The listing builds one solid part. Answer for the finished solid, in the listing's coordinates (mm). Face numbers are marked on the shaded views. A direction names the side the tool comes from. Round coordinates to 2 decimals unless told otherwise and drop trailing zeros. Write each loop counter-clockwise with the first axis right and the second up, starting at its lowest first coordinate (ties: lowest second). Pieces come first, ordered by that corner, then holes. Notation, with made-up numbers: M 14,-17.75 L 26,-17.75 A23 cw 26,-5.75 Z; hole C -9,-1 d4. An arc over 180 degrees is marked long. Write each question's results on one line, items separated by ' | '.
from build123d import *

# Parameters (mm, degrees)
F1_DEPTH       = 25
F2_R           = 20
F3_R           = 5
F5_D           = 6.7564
F5_DEPTH       = 15
F5_CSINK_D     = 13.4874
F5_CSINK_ANGLE = 82
F5_TIP         = 2.0298273432
F6_R           = 2


with BuildPart() as f1:
    # F0 (on Front) → F1 (new body)
    with BuildSketch(Plane.XZ):
        Polygon((-70.8, 12.7), (-102.55, 12.7), (-102.55, 0), (102.55, 0), (102.55, 12.7), (70.8, 12.7), (50.8, 12.7), (-50.8, 12.7), align=None)
        with BuildLine():
            ThreePointArc((70.8, 12.7), (0, 83.5), (-70.8, 12.7))
            Line((-70.8, 12.7), (-50.8, 12.7))
            ThreePointArc((-50.8, 12.7), (0, 63.5), (50.8, 12.7))
            Line((50.8, 12.7), (70.8, 12.7))
        make_face()
    extrude(amount=F1_DEPTH)

    # F2
    f2_edges = [f1.edges().sort_by_distance(p)[0] for p in [
        (50.8, -12.5, 12.7),
        (-50.8, -12.5, 12.7),
    ]]
    fillet(f2_edges, radius=F2_R)

    # F3
    f3_edges = [f1.edges().sort_by_distance(p)[0] for p in [
        (70.8, -12.5, 12.7),
        (-70.8, -12.5, 12.7),
    ]]
    fillet(f3_edges, radius=F3_R)

    # F5
    with Locations(Plane.XY.offset(12.7)):
        with Locations((89.0924562867, -12.5), (-89.0924562867, -12.5)):
            CounterSinkHole(F5_D / 2, F5_CSINK_D / 2, depth=F5_DEPTH, counter_sink_angle=F5_CSINK_ANGLE)
            with Locations((0, 0, -(F5_DEPTH + F5_TIP / 2))):  # 118° drill point
                Cone(0, F5_D / 2, F5_TIP, mode=Mode.SUBTRACT)

    # F6
    f6_edges = [f1.edges().sort_by_distance(p)[0] for p in [
        (-89.092456, -25, 12.7),
        (-72.217975, -25, 14.049721),
        (-102.55, -25, 6.35),
        (0, -25, 83.5),
        (0, -25, 0),
        (72.217975, -25, 14.049721),
        (102.55, -25, 6.35),
        (89.092456, -25, 12.7),
        (0, -25, 12.7),
        (41.585393, -25, 24.325642),
        (-41.585393, -25, 24.325642),
        (0, -25, 63.5),
        (-89.092456, 0, 12.7),
        (-72.217975, 0, 14.049721),
        (-102.55, 0, 6.35),
        (0, 0, 83.5),
        (0, 0, 0),
        (72.217975, 0, 14.049721),
        (102.55, 0, 6.35),
        (89.092456, 0, 12.7),
        (0, 0, 12.7),
        (41.585393, 0, 24.325642),
        (-41.585393, 0, 24.325642),
        (0, 0, 63.5),
    ]]
    fillet(f6_edges, radius=F6_R)


solid = f1.part
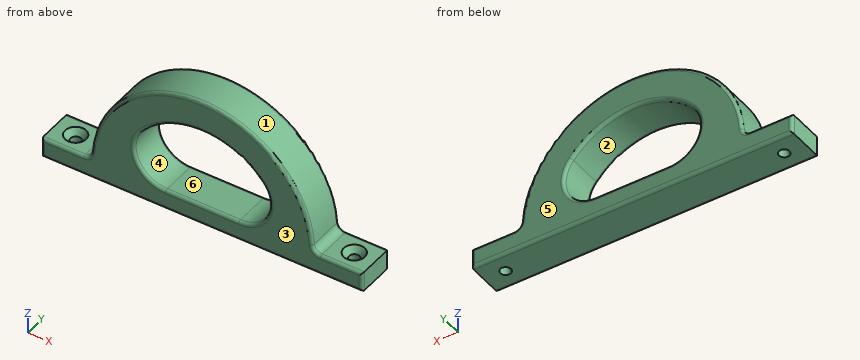
1) The mould has two halves that part along X. Classify the marked faces 1, 2, 3 and 4: +X half, -X half, draft (parallel to the pull), parting line (faces both ways), or undercut.
Return value:
face 1: parting line | face 2: undercut | face 3: draft | face 4: undercut
2) Section A-A (y = -12.5) is taken. Determine the outline of the cut face in (x, z).
Return value:
outline: M -102.55,0 L -92.47,0 L -92.47,8.83 L -95.84,12.7 L -102.55,12.7 Z; M -85.71,0 L 85.71,0 L 85.71,8.83 L 82.35,12.7 L 75.63,12.7 A5 cw 70.65,17.37 A70.8 ccw -70.65,17.37 A5 cw -75.63,12.7 L -82.35,12.7 L -85.71,8.83 Z; M 92.47,0 L 102.55,0 L 102.55,12.7 L 95.84,12.7 L 92.47,8.83 Z; hole M -38.63,45.69 A20 ccw -23.42,12.7 L 23.42,12.7 A20 ccw 38.63,45.69 A50.8 ccw Z
3) A tool of negligible diameter and unlimited length cuts with its end or side. For the marked faces 5 and 6, from which of +Z, -Z, +X, -X, +Y, -Y can it reach the whole face along a straight path? Write none if from no direction.
Return value:
face 5: +Z, -Z, +X, -X, +Y | face 6: +Y, -Y
4) Each of these flat-tipped pins is pushed along its axis until it touches: pin 1 (12 mm diameter, centred on x = -22, y = -9.5, fed in from +Z); pin 2 (8 mm diameter, centred on x = 18.5, y = -22, fed in from +Z); pin 3 (1 mm diameter, centred on y = -12, z = 47.5, fed in from -X). Where does it stop, or does it pass through?
Return value:
pin 1: z = 81.67 | pin 2: z = 82 | pin 3: x = -61.94
5) Section B-B (x = -79) is taken. Determine the outline of the cut face in (y, z), then the cut area to 3 significant figures.
Return value:
outline: M -25,2 A2 ccw -23,0 L -2,0 A2 ccw 0,2 L 0,10.7 A2 ccw -2,12.7 L -23,12.7 A2 ccw -25,10.7 Z | area: 314 mm²
6) Find the intervals of material crossed by line 1 (X direction, y = -12.5, z = 4.5); line 2 (Z direction, x = 78.5, y = -2.75); line 3 (X direction, y = -11.75, z = 3), in increasing order.
Return value:
line 1: -102.55 to -92.47, -85.71 to 85.71, 92.47 to 102.55 | line 2: 0 to 12.7 | line 3: -102.55 to -92.39, -85.8 to 85.8, 92.39 to 102.55
7) Section C-C (x = 0) is taken. Determine the outline of the cut face in (y, z), then the cut area to 3 significant figures.
Return value:
outline: M -25,2 A2 ccw -23,0 L -2,0 A2 ccw 0,2 L 0,10.7 A2 ccw -2,12.7 L -23,12.7 A2 ccw -25,10.7 Z; M -25,65.5 A2 ccw -23,63.5 L -2,63.5 A2 ccw 0,65.5 L 0,81.5 A2 ccw -2,83.5 L -23,83.5 A2 ccw -25,81.5 Z | area: 811 mm²
